from build123d import *

# Parameters (mm, degrees)
SKETCH026_W     = 36.83
SKETCH026_H     = 68.58
PAD014_DEPTH    = 2.54
SKETCH027_W     = 36.83
SKETCH027_H     = 68.58
SKETCH027_W_2   = 31.75
SKETCH027_H_2   = 62.23
PAD015_DEPTH    = 12.065
SKETCH028_R     = 3.175
PAD016_DEPTH    = 12.065
SKETCH029_R     = 1.143
POCKET009_DEPTH = 9.525
SKETCH030_R     = 3.175
PAD017_DEPTH    = 15.875
SKETCH031_R     = 1.143
POCKET010_DEPTH = 9.525
PAD018_DEPTH    = 2.54
SKETCH033_R     = 2.794
SKETCH033_R_2   = 5.08
POCKET011_DEPTH = 5.08
POCKET012_DEPTH = 12.065
SKETCH035_W     = 5.08
SKETCH035_H     = 1.143
SKETCH035_W_2   = 29.21
PAD019_DEPTH    = 1.27
POCKET013_DEPTH = 1.524
FILLET_R        = 1.27


with BuildPart() as part:
    # Sketch026 → Pad014 (new body)
    with BuildSketch(Plane.XY):
        with Locations((15.875, 31.75)):
            Rectangle(SKETCH026_W, SKETCH026_H)
    extrude(amount=PAD014_DEPTH)

    # Sketch027 (on Face5 of Pad014) → Pad015 (join)
    with BuildSketch(Plane(origin=(0, 0, 0), x_dir=(1, 0, 0), z_dir=(0, 0, -1))):
        with Locations((15.875, -31.75)):
            Rectangle(SKETCH027_W, SKETCH027_H)
        with Locations((15.875, -31.115)):
            Rectangle(SKETCH027_W_2, SKETCH027_H_2, mode=Mode.SUBTRACT)
    extrude(amount=PAD015_DEPTH)

    # Sketch028 (on Face15 of Pad015) → Pad016 (join)
    with BuildSketch(Plane(origin=(0, 0, 0), x_dir=(1, 0, 0), z_dir=(0, 0, -1))):
        with Locations((7.62, -50.8)):
            Circle(SKETCH028_R)
        with Locations((24.13, -50.8)):
            Circle(SKETCH028_R)
    extrude(amount=PAD016_DEPTH)

    # Sketch029 (on Face18 of Pad016) → Pocket009 (cut)
    with BuildSketch(Plane(origin=(0, 0, -12.065), x_dir=(1, 0, 0), z_dir=(0, 0, -1))):
        with Locations((7.62, -50.8)):
            Circle(SKETCH029_R)
        with Locations((24.13, -50.8)):
            Circle(SKETCH029_R)
    extrude(amount=-POCKET009_DEPTH, mode=Mode.SUBTRACT)

    # Sketch030 (on Face15 of Pocket009) → Pad017 (join)
    with BuildSketch(Plane(origin=(0, 0, 0), x_dir=(1, 0, 0), z_dir=(0, 0, -1))):
        with Locations((7.62, -22.225)):
            Circle(SKETCH030_R)
    extrude(amount=PAD017_DEPTH)

    # Sketch031 (on Face19 of Pad017) → Pocket010 (cut)
    with BuildSketch(Plane(origin=(0, 0, -15.875), x_dir=(1, 0, 0), z_dir=(0, 0, -1))):
        with Locations((7.62, -22.225)):
            Circle(SKETCH031_R)
    extrude(amount=-POCKET010_DEPTH, mode=Mode.SUBTRACT)

    # Sketch032 (on Face4 of Pocket010) → Pad018 (join)
    with BuildSketch(Plane.XZ.offset(2.54)):
        Polygon((2.794, -12.065), (12.446, -12.065), (11.43, -13.335), (7.62, -13.335), (3.81, -13.335), align=None)
    extrude(amount=-PAD018_DEPTH)

    # Sketch033 (on Face4 of Pad018) → Pocket011 (cut)
    with BuildSketch(Plane.XZ.offset(2.54)):
        with Locations((7.62, -13.335)):
            Circle(SKETCH033_R)
        with Locations((23.495, -12.065)):
            Circle(SKETCH033_R_2)
    extrude(amount=-POCKET011_DEPTH, mode=Mode.SUBTRACT)

    # Sketch034 (on Face9 of Pocket011) → Pocket012 (cut)
    with BuildSketch(Plane(origin=(0, 0, -12.065), x_dir=(1, 0, 0), z_dir=(0, 0, -1))):
        Polygon((1.27, -62.23), (1.27, -63.373), (0, -63.373), (0, -64.897), (1.27, -64.897), (1.27, -66.04), (30.48, -66.04), (30.48, -64.897), (31.75, -64.897), (31.75, -63.373), (30.48, -63.373), (30.48, -62.23), align=None)
    extrude(amount=-POCKET012_DEPTH, mode=Mode.SUBTRACT)

    # Sketch035 (on Face17 of Pocket012) → Pad019 (join)
    with BuildSketch(Plane(origin=(0, 0, 0), x_dir=(1, 0, 0), z_dir=(0, 0, -1))):
        with Locations((3.81, -62.8015)):
            Rectangle(SKETCH035_W, SKETCH035_H)
        with Locations((15.875, -65.4685)):
            Rectangle(SKETCH035_W_2, SKETCH035_H)
        with Locations((27.94, -62.8015)):
            Rectangle(SKETCH035_W, SKETCH035_H)
    extrude(amount=PAD019_DEPTH)

    # Sketch036 (on Face15 of Pad019) → Pocket013 (cut)
    with BuildSketch(Plane(origin=(0, 0, -12.065), x_dir=(1, 0, 0), z_dir=(0, 0, -1))):
        Polygon((-1.397, 1.397), (-1.397, -63.627), (33.147, -63.627), (33.147, 1.397), (12.446, 1.397), (12.446, 0), (31.75, 0), (31.75, -62.23), (0, -62.23), (0, 0), (2.794, 0), (2.794, 1.397), align=None)
    extrude(amount=-POCKET013_DEPTH, mode=Mode.SUBTRACT)

    # Fillet
    fillet_edges = [part.edges().sort_by_distance(p)[0] for p in [
        (34.29, 31.75, 2.54),
        (15.875, 66.04, 2.54),
        (-2.54, 31.75, 2.54),
        (15.875, -2.54, 2.54),
        (34.29, -2.54, 1.27),
        (34.29, -2.54, -6.0325),
        (34.29, 66.04, 1.27),
        (34.29, 66.04, -6.0325),
        (-2.54, 66.04, -6.0325),
        (-2.54, 66.04, 1.27),
        (-2.54, -2.54, -6.0325),
        (-2.54, -2.54, 1.27),
    ]]
    fillet(fillet_edges, radius=FILLET_R)


with BuildPart() as part_1:
    # Body020 placement: moved
    add(part.part.moved(Location((0, 0, 15.875))))


solid = part_1.part
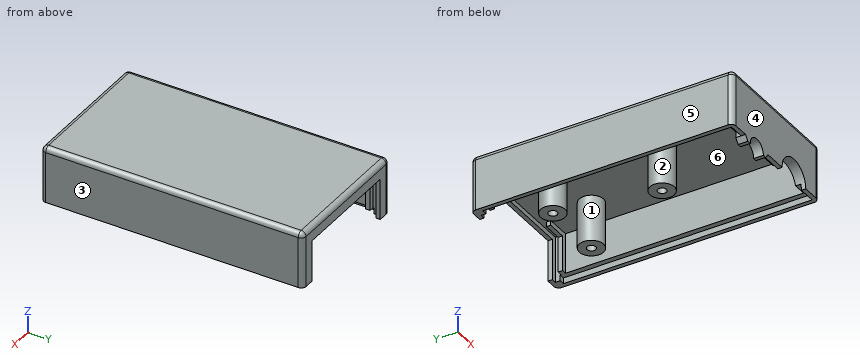
Source: CAD feature listing. Evaluate the final solid. Frame: model axes, mm. Face numbers are marked on the shaded views. A direction names the side the tool comes from. Coordinates: 2 decimals unless noted, no trailing zeros. Loops run counter-clockwise (first coordinate to the right, second up) from the corner with the lowest first, then second, coordinate; pieces in that order, holes last. Notation, with made-up numbers: (17.25, 88.5) -> (29.25, 88.5) arc R28 ccw to (29.25, 123.5) -> close; hole circle Ø3 at (70.5, 58.25). An arc over 180 degrees is marked (long way). Answer in a Markdown table with one row per item. Add a question column.
Q1. Contact query for flat-ended pins moving along their axis: pin 1 Ø1.5 at (x, y) = (15, -0.5) entering from -Z; pin 2 Ø4 at (x, z) = (5, 9) entering from +Y; pin 3 Ø8 at (x, z) = (2, 10) entering from +Y; pin 4 Ø0.6 at (x, y) = (17, 65.5) entering from -Z (3 decimals). Output: stop coordinate, or through.
Q2. Section B-B on y = 13.5. Return the cut outline in (x, z) (3 decimals).
Q3. Ray query, line 1 along X through (y, z) = (50.8, 9) (3 decimals); line 2 along Y through (x, z) = (24.13, 9.5) (3 decimals); line 3 along Y through (x, z) = (7.62, 4.5) (3 decimals). Return the intervals inside material, ascending.
Q4. Section D-D on x = 22. Return the cut outline in (y, z) (3 decimals), and give its area (3 significant figures).
Q5. Reachability of the marked faces 5 and 6 from +Z, -Z, +X, -X, +Y, -Y: full face, straight path, thin tool, end or side. Return the list, or none.
Q6. Pull-direction query (X, two-part tool) for the marked faces 1, 2, 3 and 4; classes: pulls with the +X half, pulls with the -X half, needs draft (parallel to the pull), parting line crosses it, or undercut.
Q7. Section A-A on z = 6.25. Give the number of separate pieces and of enclosed holes in the cut face, and give its area (3 significant figures).
Computed values:
| question | item | result |
|---|---|---|
| 1 | pin 1 | stops at z = 5.33 |
| 1 | pin 2 | stops at y = 53.91 |
| 1 | pin 3 | stops at y = 66.04 |
| 1 | pin 4 | stops at z = 14.605 |
| 2 | outline | (-2.54, 3.81) -> (-1.397, 3.81) -> (-1.397, 5.334) -> (0, 5.334) -> (0, 15.875) -> (31.75, 15.875) -> (31.75, 5.334) -> (33.147, 5.334) -> (33.147, 3.81) -> (34.29, 3.81) -> (34.29, 17.145) arc R1.27 ccw to (33.02, 18.415) -> (-1.27, 18.415) arc R1.27 ccw to (-2.54, 17.145) -> close |
| 3 | line 1 | x = -2.54 to 0, 4.445 to 6.477, 8.763 to 10.795, 20.955 to 22.987, 25.273 to 27.305, 31.75 to 34.29 |
| 3 | line 2 | y = -2.54 to 0, 47.625 to 49.657, 51.943 to 53.975 |
| 3 | line 3 | y = 19.05 to 21.082, 23.368 to 25.4, 47.625 to 49.657, 51.943 to 53.975 |
| 4 | outline | (-2.54, 8.665) -> (0, 8.665) -> (0, 15.875) -> (48.445, 15.875) -> (48.445, 3.81) -> (53.155, 3.81) -> (53.155, 15.875) -> (64.897, 15.875) -> (64.897, 14.605) -> (66.04, 14.605) -> (66.04, 17.145) arc R1.27 ccw to (64.77, 18.415) -> (-1.27, 18.415) arc R1.27 ccw to (-2.54, 17.145) -> close |
| 4 | area | 250 mm^2 |
| 5 | face 5 | +Z, -Z, -X, +Y, -Y |
| 5 | face 6 | -Z |
| 6 | face 1 | undercut |
| 6 | face 2 | undercut |
| 6 | face 3 | pulls with the +X half |
| 6 | face 4 | needs draft |
| 7 | separate pieces | 5 |
| 7 | enclosed holes | 3 |
| 7 | area | 494 mm^2 |
